from build123d import *

# Parameters (mm, degrees)
BOSS_EXTRUDE1_DEPTH                                = 11.7
SKETCH12_W                                         = 26.901846944
SKETCH12_H                                         = 2.5
CUT_EXTRUDE6_DEPTH                                 = 43.3
SKETCH13_W                                         = 26.901846944
SKETCH13_H                                         = 2.5
CUT_EXTRUDE7_DEPTH                                 = 43.3
SKETCH14_R                                         = 3.25
CUT_EXTRUDE8_DEPTH                                 = 3
SKETCH15_R                                         = 2.5
CUT_EXTRUDE9_DEPTH                                 = 9.7
CBORE_FOR_M2_5_PAN_HEAD_MACHINE_SCREW1_D           = 2.9
CBORE_FOR_M2_5_PAN_HEAD_MACHINE_SCREW1_CBORE_D     = 6
CBORE_FOR_M2_5_PAN_HEAD_MACHINE_SCREW1_CBORE_DEPTH = 2.1


with BuildPart() as part:
    # Sketch1 → Boss-Extrude1 (new body)
    with BuildSketch(Plane(origin=(0, 0, 0), x_dir=(1, 0, 0), z_dir=(0, 1, 0))):
        Polygon((-21.15, 16.750923472), (-16.750923472, 21.15), (16.750923472, 21.15), (21.15, 16.750923472), (21.15, -16.750923472), (16.750923472, -21.15), (-16.750923472, -21.15), (-21.15, -16.750923472), align=None)
    extrude(amount=BOSS_EXTRUDE1_DEPTH)

    # Sketch12 → Cut-Extrude6 (cut, through all)
    with BuildSketch(Plane(origin=(21.15, 0, 0), x_dir=(0, 0, -1), z_dir=(1, 0, 0))):
        with Locations((0, 10.45)):
            Rectangle(SKETCH12_W, SKETCH12_H)
    extrude(amount=-CUT_EXTRUDE6_DEPTH, mode=Mode.SUBTRACT)

    # Sketch13 → Cut-Extrude7 (cut, through all)
    with BuildSketch(Plane.XY.offset(21.15)):
        with Locations((0, 10.45)):
            Rectangle(SKETCH13_W, SKETCH13_H)
    extrude(amount=-CUT_EXTRUDE7_DEPTH, mode=Mode.SUBTRACT)

    # Sketch14 → Cut-Extrude8 (cut)
    with BuildSketch(Plane.XZ):
        Circle(SKETCH14_R)
    extrude(amount=-CUT_EXTRUDE8_DEPTH, mode=Mode.SUBTRACT)

    # Sketch15 → Cut-Extrude9 (cut, through all)
    with BuildSketch(Plane.XZ.offset(-3)):
        Circle(SKETCH15_R)
    extrude(amount=-CUT_EXTRUDE9_DEPTH, mode=Mode.SUBTRACT)

    # CBORE for M2.5 Pan Head Machine Screw1 (through all)
    with Locations(Plane(origin=(0, 0, 0), x_dir=(-1, 0, 0), z_dir=(0, -1, 0))):
        with Locations((15, -15), (-15, -15), (-15, 15), (15, 15)):
            CounterBoreHole(CBORE_FOR_M2_5_PAN_HEAD_MACHINE_SCREW1_D / 2, CBORE_FOR_M2_5_PAN_HEAD_MACHINE_SCREW1_CBORE_D / 2, CBORE_FOR_M2_5_PAN_HEAD_MACHINE_SCREW1_CBORE_DEPTH)


solid = part.part
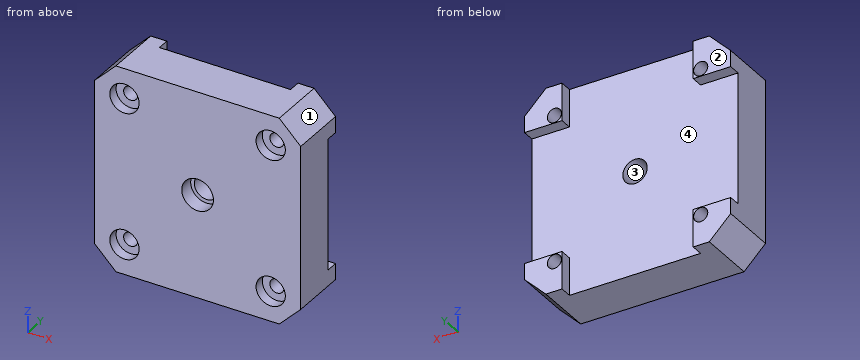
Part model, mm, in its own coordinate system. Face numbers are marked on the shaded views. Give positions to 0.01 mm unless a question says otherwise; leave off trailing zeros. Order: outer loops, then holes, each group sorted by start corner. A loop starts at its lowest first (then second) coordinate and runs counter-clockwise, first axis right, second up. Notation, with made-up numbers: (9.5, 30.25) - (19.5, 30.25) arc R24 cw to (19.5, 52.25) - close; hole circle Ø2 at (4, 22). An arc over 180 degrees is marked (long way). Use a Markdown table: item, result.
1) Saw through at B-B on z = 0. List the corners of the cut face in (x, y), plus the area to 3 significant figures.
Checked values:
| item | result |
|---|---|
| outline | (-21.15, 0) - (-3.25, 0) - (-3.25, 3) - (-2.5, 3) - (-2.5, 9.2) - (-21.15, 9.2) - close; (2.5, 3) - (3.25, 3) - (3.25, 0) - (21.15, 0) - (21.15, 9.2) - (2.5, 9.2) - close |
| area | 339 mm² |
2) Probe L1, parallel to X at y = 0.45, z = 15; L2, parallel to Z at x = -15, y = 4.75; L3, parallel to Z at x = 16, y = 5.25. List the from-to ranges inside material, lowest first. Write a range as from..to.
Checked values:
| item | result |
|---|---|
| L1 | -21.15..-18, -12..12, 18..21.15 |
| L2 | -21.15..-16.45, -13.55..13.55, 16.45..21.15 |
| L3 | -21.15..-16.05, -13.95..13.95, 16.05..21.15 |
3) Flat gauge pins, fed straight in: P1, Ø1, axis at x = 2.5, z = 10, coming from the +Y side; P2, Ø0.8, axis at x = 18, y = 10.5, coming from the -Z side; P3, Ø2, axis at y = 11, z = -18, coming from the -X side. Where does each tip first touch, or does it go through?
Checked values:
| item | result |
|---|---|
| P1 | y = 9.2 |
| P2 | z = -20.3 |
| P3 | x = -20.9 |
4) Saw through at C-C on x = 0. List the corners of the cut face in (y, z), plus the area to 3 significant figures.
Checked values:
| item | result |
|---|---|
| outline | (0, -21.15) - (9.2, -21.15) - (9.2, -2.5) - (3, -2.5) - (3, -3.25) - (0, -3.25) - close; (0, 3.25) - (3, 3.25) - (3, 2.5) - (9.2, 2.5) - (9.2, 21.15) - (0, 21.15) - close |
| area | 339 mm² |
5) Saw through at A-A on y = 10. List the corners of the cut face in (x, z), plus the area to 3 significant figures.
Checked values:
| item | result |
|---|---|
| outline | (-21.15, -16.75) - (-16.75, -21.15) - (-13.45, -21.15) - (-13.45, -13.45) - (-21.15, -13.45) - close; (-21.15, 13.45) - (-13.45, 13.45) - (-13.45, 21.15) - (-16.75, 21.15) - (-21.15, 16.75) - close; (13.45, -21.15) - (16.75, -21.15) - (21.15, -16.75) - (21.15, -13.45) - (13.45, -13.45) - close; (13.45, 13.45) - (21.15, 13.45) - (21.15, 16.75) - (16.75, 21.15) - (13.45, 21.15) - close; hole circle Ø2.9 at (-15, -15); hole circle Ø2.9 at (-15, 15); hole circle Ø2.9 at (15, -15); hole circle Ø2.9 at (15, 15) |
| area | 172 mm² |
6) Two-plate mould, pull along Z, no slides. Class the marked faces 1, 2, 3 and 4: +Z half, -Z half, draft (parallel to the pull), parting line (faces both ways), or undercut.
Checked values:
| item | result |
|---|---|
| face 1 | +Z half |
| face 2 | draft |
| face 3 | undercut |
| face 4 | undercut |
7) Saw through at D-D on z = -15. List the corners of the cut face in (x, y).
Checked values:
| item | result |
|---|---|
| outline | (-21.15, 0) - (-18, 0) - (-18, 2.1) - (-16.45, 2.1) - (-16.45, 11.7) - (-21.15, 11.7) - close; (-13.55, 2.1) - (-12, 2.1) - (-12, 0) - (12, 0) - (12, 2.1) - (13.55, 2.1) - (13.55, 11.7) - (13.45, 11.7) - (13.45, 9.2) - (-13.45, 9.2) - (-13.45, 11.7) - (-13.55, 11.7) - close; (16.45, 2.1) - (18, 2.1) - (18, 0) - (21.15, 0) - (21.15, 11.7) - (16.45, 11.7) - close |
